from build123d import *

# Parameters (mm, degrees)
SKETCH1_W                   = 30
SKETCH1_H                   = 10
BASE_FLANGE1_DEPTH          = 1.5
F_3_0MM_PRESS_DOWEL_HOLE1_D = 3


# Sheet-metal steps are written as plain solids
with BuildPart() as part:
    # Sketch1 → Base-Flange1 (new body)
    with BuildSketch(Plane(origin=(0, 0, 0), x_dir=(1, 0, 0), z_dir=(0, 1, 0))):
        with Locations((15, 5)):
            Rectangle(SKETCH1_W, SKETCH1_H)
    extrude(amount=-BASE_FLANGE1_DEPTH)

    # Ø3.0mm Press Dowel Hole1 (through all)
    with Locations(Plane(origin=(0, 0, 0), x_dir=(1, 0, 0), z_dir=(0, 1, 0))):
        with Locations((10, 5)):
            Hole(F_3_0MM_PRESS_DOWEL_HOLE1_D / 2)


solid = part.part
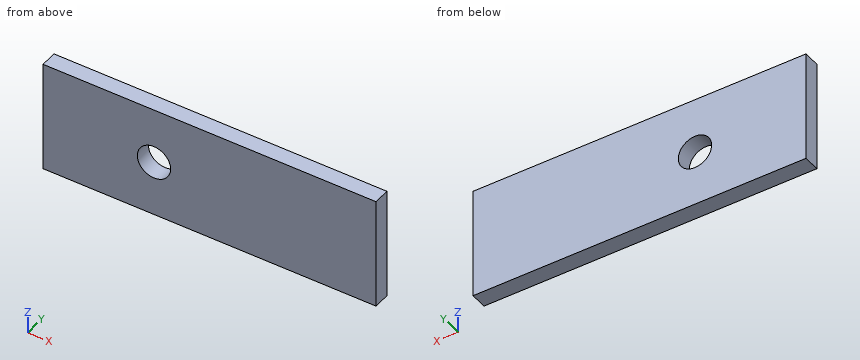
Can you work these out from the model? Positions are in its coordinate system, mm. Coordinates: 2 decimals unless noted, no trailing zeros. Order: outer loops, then holes, each group sorted by start corner. A loop starts at its lowest first (then second) coordinate and runs counter-clockwise, first axis right, second up. Notation, with made-up numbers: (50, -19) -> (107, -19) arc R25 ccw to (107, 5) -> close; hole circle Ø7 at (1, -23). An arc over 180 degrees is marked (long way). Use one line per item in the form item = value.
Q1. Imagine slicing it at B-B, the plane x = 10. List the corners of the cut face in (y, z) for me, then the cut area to 3 significant figures.
From the geometry:
outline = (-1.5, -10) -> (0, -10) -> (0, -6.5) -> (-1.5, -6.5) -> close; (-1.5, -3.5) -> (0, -3.5) -> (0, 0) -> (-1.5, 0) -> close
area = 10.5 mm²
Q2. Imagine slicing it at A-A, the plane z = -5. List the corners of the cut face in (x, y) for me.
From the geometry:
outline = (0, -1.5) -> (8.5, -1.5) -> (8.5, 0) -> (0, 0) -> close; (11.5, -1.5) -> (30, -1.5) -> (30, 0) -> (11.5, 0) -> close
Q3. I need wall thicknesses on L1, parallel to X at y = -0.5, z = -5; L2, parallel to Z at x = 10, y = -0.45; L3, parallel to X at y = -0.95, z = -5.5. Which ranges of each line are inside material? Lowest first, please.
From the geometry:
L1 = 0 to 8.5, 11.5 to 30
L2 = -10 to -6.5, -3.5 to 0
L3 = 0 to 8.59, 11.41 to 30
Q4. Imagine slicing it at C-C, the plane y = -1.2. List the corners of the cut face in (x, z) for me, then the cut area to 3 significant figures.
From the geometry:
outline = (0, -10) -> (30, -10) -> (30, 0) -> (0, 0) -> close; hole circle Ø3 at (10, -5)
area = 293 mm²
